Here's how the part is built. I have some questions about the finished solid (model axes, mm). A direction names the side the tool comes from. Round coordinates to 2 decimals unless told otherwise and drop trailing zeros. Order: outer loops, then holes, each group sorted by start corner. A loop starts at its lowest first (then second) coordinate and runs counter-clockwise, first axis right, second up. Notation, with made-up numbers: (48.25, 82.25) -> (69.25, 82.25) arc R29 cw to (69.25, 103.25) -> close; hole circle Ø6 at (-3, 69.25). An arc over 180 degrees is marked (long way). Use a Markdown table: item, result. Add a question column.
(1) I want a section at A-A, the plane y = 0. Give the number of separate pieces and of enclosed holes in the cut face, then the cut area to 3 significant figures.
(2) On a 3-axis mill with a long thin cutter (end or side, diameter ignored), from which of +Z, -Z, +X, -X, +Y, -Y can I reach the whole of each face in a straight line? I mean faces 1 (the face through (14.5, 0, -102.5)), 2 (the face through (16, -3, -105)), 3 (the face through (1.4, -14.8, -104)). Say none if no direction works.
(3) If I drill on probe 1 along X at (y, z) = (0, -109.55); probe 2 along X at (y, z) = (16, -102), over which ranges is the centre line in solid material (lowest first)?
(4) I want a section at C-C, the plane z = -105. Please give me the cut outline in (x, y), then the cut area to 3 significant figures.
(5) Thinking about a two-plate mould opening in X: for faces 4 (the face through (-14.8, -1.4, -104)), 5 (the face through (14.5, 0, -109)), which applies, pulls with the +X half, pulls with the -X half, needs draft (parallel to the pull), parting line crosses it, or undercut?
(6) I'm going to push flat-ended pins straight in: P1, Ø2, axis at x = -15.5, z = -110.5, coming from the -Y side (3 decimals); P2, Ø2, axis at y = -14, z = -105, coming from the +X side; P3, Ø4, axis at x = 14, z = -109.5, coming from the -Y side. Where does each tip first touch, or does it pass through?
from build123d import *

# Parameters (mm, degrees)
BOX106_W                    = 10
BOX106_H                    = 6
BOX106_DEPTH                = 2
BOX105_W                    = 10
BOX105_H                    = 6
BOX105_DEPTH                = 2
BOX107_W                    = 10
BOX107_H                    = 6
BOX107_DEPTH                = 2
BOX104_W                    = 10
BOX104_H                    = 6
BOX104_DEPTH                = 2
CYLINDER279_R               = 1.5
CYLINDER279_DEPTH           = 16
CYLINDER279_PLACEMENT_ANGLE = 67.5
CYLINDER277_R               = 1.5
CYLINDER277_DEPTH           = 16
CYLINDER277_PLACEMENT_ANGLE = 22.5
CYLINDER278_R               = 1.5
CYLINDER278_DEPTH           = 16
CYLINDER278_PLACEMENT_ANGLE = 112.5
CYLINDER276_R               = 1.5
CYLINDER276_DEPTH           = 16
CYLINDER276_PLACEMENT_ANGLE = 202.5
TUBE031_R                   = 20
TUBE031_R_2                 = 12
TUBE031_DEPTH               = 11
CHAMFER004_SIZE             = 1


with BuildPart() as krychle106:
    # Box106 → Box106 (new body)
    with BuildSketch(Plane(origin=(3, 11, 6), x_dir=(0, 1, 0), z_dir=(0, 0, 1))):
        with Locations((5, 3)):
            Rectangle(BOX106_W, BOX106_H)
    extrude(amount=BOX106_DEPTH)


with BuildPart() as krychle105:
    # Box105 → Box105 (new body)
    with BuildSketch(Plane(origin=(-11, 3, 6), x_dir=(-1, 0, 0), z_dir=(0, 0, 1))):
        with Locations((5, 3)):
            Rectangle(BOX105_W, BOX105_H)
    extrude(amount=BOX105_DEPTH)


with BuildPart() as krychle107:
    # Box107 → Box107 (new body)
    with BuildSketch(Plane(origin=(-3, -11, 6), x_dir=(0, -1, 0), z_dir=(0, 0, 1))):
        with Locations((5, 3)):
            Rectangle(BOX107_W, BOX107_H)
    extrude(amount=BOX107_DEPTH)


with BuildPart() as compound232:
    # Box104 → Box104 (new body)
    with BuildSketch(Plane(origin=(11, -3, 6), x_dir=(1, 0, 0), z_dir=(0, 0, 1))):
        with Locations((5, 3)):
            Rectangle(BOX104_W, BOX104_H)
    extrude(amount=BOX104_DEPTH)

    # Compound232: union Krychle106, Krychle105, Krychle107
    add(krychle106.part)
    add(krychle105.part)
    add(krychle107.part)


with BuildPart() as compound232_1:
    # Compound232 placement: moved
    add(compound232.part.moved(Location((0, 0, -111))))


with BuildPart() as obj1:
    # Cylinder279 → Cylinder279 (new body)
    with BuildSketch(Plane.XY):
        Circle(CYLINDER279_R)
    extrude(amount=CYLINDER279_DEPTH)


with BuildPart() as obj1_1:
    # Cylinder279 placement: moved
    add(obj1.part.moved(Location((0, 16, 2))).rotate(Axis((0, 16, 2), (0, 0, -1)), CYLINDER279_PLACEMENT_ANGLE))


with BuildPart() as obj2:
    # Cylinder277 → Cylinder277 (new body)
    with BuildSketch(Plane.XY):
        Circle(CYLINDER277_R)
    extrude(amount=CYLINDER277_DEPTH)


with BuildPart() as obj2_1:
    # Cylinder277 placement: moved
    add(obj2.part.moved(Location((-16, 0, 2))).rotate(Axis((-16, 0, 2), (0, 0, 1)), CYLINDER277_PLACEMENT_ANGLE))


with BuildPart() as obj3:
    # Cylinder278 → Cylinder278 (new body)
    with BuildSketch(Plane.XY):
        Circle(CYLINDER278_R)
    extrude(amount=CYLINDER278_DEPTH)


with BuildPart() as obj3_1:
    # Cylinder278 placement: moved
    add(obj3.part.moved(Location((0, -16, 2))).rotate(Axis((0, -16, 2), (0, 0, 1)), CYLINDER278_PLACEMENT_ANGLE))


with BuildPart() as compound234:
    # Cylinder276 → Cylinder276 (new body)
    with BuildSketch(Plane.XY):
        Circle(CYLINDER276_R)
    extrude(amount=CYLINDER276_DEPTH)


with BuildPart() as compound234_1:
    # Cylinder276 placement: moved
    add(compound234.part.moved(Location((16, 0, 2))).rotate(Axis((16, 0, 2), (0, 0, 1)), CYLINDER276_PLACEMENT_ANGLE))

    # Compound234: union obj1, obj2, obj3
    add(obj1_1.part)
    add(obj2_1.part)
    add(obj3_1.part)


with BuildPart() as compound234_2:
    # Compound234 placement: moved
    add(compound234_1.part.moved(Location((0, 0, -117))))


with BuildPart() as chamfer004:
    # Tube031 → Tube031 (new body)
    with BuildSketch(Plane.XY.offset(-111)):
        Circle(TUBE031_R)
        Circle(TUBE031_R_2, mode=Mode.SUBTRACT)
    extrude(amount=TUBE031_DEPTH)

    # Cut123: cut Compound234
    add(compound234_2.part, mode=Mode.SUBTRACT)

    # Cut126: cut Compound232
    add(compound232_1.part, mode=Mode.SUBTRACT)

    # Chamfer004
    chamfer004_edges = [chamfer004.edges().sort_by_distance(p)[0] for p in [
        (-20, 0, -111),
    ]]
    chamfer(chamfer004_edges, length=CHAMFER004_SIZE)


with BuildPart() as chamfer004_1:
    # Chamfer004 placement: moved
    add(chamfer004.part.moved(Location((0, 0, -1))))


solid = chamfer004_1.part
Taken from the geometry:
| question | item | result |
|---|---|---|
| 1 | separate pieces | 8 |
| 1 | enclosed holes | 0 |
| 1 | area | 89.0 mm2 |
| 2 | face 1 | +Z, -Z |
| 2 | face 2 | +X, -X |
| 2 | face 3 | +Y, -Y |
| 3 | probe 1 | x = -20 to -17.5, -14.5 to -12, 12 to 14.5, 17.5 to 20 |
| 3 | probe 2 | x = -12 to -1.5, 1.5 to 12 |
| 4 | outline | (-19.77, -3) arc R20 ccw to (-3, -19.77) -> (-3, -11.62) arc R12 cw to (-11.62, -3) -> close; (-19.77, 3) -> (-11.62, 3) arc R12 cw to (-3, 11.62) -> (-3, 19.77) arc R20 ccw to start; (3, -19.77) arc R20 ccw to (19.77, -3) -> (11.62, -3) arc R12 cw to (3, -11.62) -> close; (3, 11.62) arc R12 cw to (11.62, 3) -> (19.77, 3) arc R20 ccw to (3, 19.77) -> close |
| 4 | area | 611 mm2 |
| 5 | face 4 | needs draft |
| 5 | face 5 | undercut |
| 6 | P1 | stops at y = -13.775 |
| 6 | P2 | stops at x = 15.2 |
| 6 | P3 | stops at y = -16 |
